```python
from build123d import *

# Parameters (mm, degrees)
F0_W     = 31.8
F0_H     = 15.8
F0_W_2   = 29.4
F0_H_2   = 13.4
F0_R     = 3.25
F0_R_2   = 2.4
F1_DEPTH = 9.6
F2_DEPTH = 7.9
F3_R     = 2.4
F4_DEPTH = 1.7
F5_W     = 0.6
F5_H     = 0.3
F5_W_2   = 0.3
F5_H_2   = 0.6
F6_DEPTH = 7.9


# Not quite as in the source:
# - a feature names something its author has since deleted; it is built from what else it names


with BuildPart() as f1:
    # F0 (on Top) → F1 (new body)
    with BuildSketch(Plane.XY):
        Rectangle(F0_W, F0_H)
        Rectangle(F0_W_2, F0_H_2, mode=Mode.SUBTRACT)
        Rectangle(F0_W_2, F0_H_2)
        with Locations((-8, 0)):
            Circle(F0_R, mode=Mode.SUBTRACT)
        Circle(F0_R, mode=Mode.SUBTRACT)
        with Locations((8, 0)):
            Circle(F0_R, mode=Mode.SUBTRACT)
        with Locations((-8, 0)):
            Circle(F0_R)
        with Locations((-8, 0)):
            Circle(F0_R_2, mode=Mode.SUBTRACT)
        Circle(F0_R)
        Circle(F0_R_2, mode=Mode.SUBTRACT)
        with Locations((8, 0)):
            Circle(F0_R)
        with Locations((8, 0)):
            Circle(F0_R_2, mode=Mode.SUBTRACT)
        with Locations((-8, 0)):
            Circle(F0_R_2)
        Circle(F0_R_2)
        with Locations((8, 0)):
            Circle(F0_R_2)
    extrude(amount=F1_DEPTH)

    # F0 (on Top) → F2 (cut)
    with BuildSketch(Plane.XY):
        Rectangle(F0_W_2, F0_H_2)
        with Locations((-8, 0)):
            Circle(F0_R, mode=Mode.SUBTRACT)
        Circle(F0_R, mode=Mode.SUBTRACT)
        with Locations((8, 0)):
            Circle(F0_R, mode=Mode.SUBTRACT)
        with Locations((-8, 0)):
            Circle(F0_R_2)
        with Locations((8, 0)):
            Circle(F0_R_2)
        Circle(F0_R_2)
    extrude(amount=F2_DEPTH, mode=Mode.SUBTRACT)

    # F3 (on face) → F4 (join)
    with BuildSketch(Plane.XY.offset(9.6)):
        with Locations((-12, 4)):
            Circle(F3_R)
        with Locations((-12, -4)):
            Circle(F3_R)
        with Locations((-4, 4)):
            Circle(F3_R)
        with Locations((-4, -4)):
            Circle(F3_R)
        with Locations((4, 4)):
            Circle(F3_R)
        with Locations((4, -4)):
            Circle(F3_R)
        with Locations((12, 4)):
            Circle(F3_R)
        with Locations((12, -4)):
            Circle(F3_R)
    extrude(amount=F4_DEPTH)

    # F5 (on Top) → F6 (join, through all)
    with BuildSketch(Plane.XY):
        with Locations((-12, -6.55)):
            Rectangle(F5_W, F5_H)
        with Locations((-4, -6.55)):
            Rectangle(F5_W, F5_H)
        with Locations((-14.55, -4)):
            Rectangle(F5_W_2, F5_H_2)
        with Locations((4, -6.55)):
            Rectangle(F5_W, F5_H)
        with Locations((12, -6.55)):
            Rectangle(F5_W, F5_H)
        with Locations((14.55, -4)):
            Rectangle(F5_W_2, F5_H_2)
        with Locations((-4, 6.55)):
            Rectangle(F5_W, F5_H)
        with Locations((14.55, 4)):
            Rectangle(F5_W_2, F5_H_2)
        with Locations((12, 6.55)):
            Rectangle(F5_W, F5_H)
        with Locations((-12, 6.55)):
            Rectangle(F5_W, F5_H)
        with Locations((-14.55, 4)):
            Rectangle(F5_W_2, F5_H_2)
        with Locations((4, 6.55)):
            Rectangle(F5_W, F5_H)
    extrude(amount=F6_DEPTH)


solid = f1.part
```
Geometry check sheet. Reference: the model listing, model coordinates, mm. A direction names the side the tool comes from. Round coordinates to 2 decimals unless told otherwise and drop trailing zeros. Order: outer loops, then holes, each group sorted by start corner. A loop starts at its lowest first (then second) coordinate and runs counter-clockwise, first axis right, second up. Notation, with made-up numbers: M -8.5,70 L 34.5,70 A29 ccw 34.5,106 Z; hole C 13,45.5 d2. An arc over 180 degrees is marked long. Answer as CSV lines item,"result".
1) Tool access check on faces 1 (the face through (-14.398, 4.106, 10.438)), 2 (the face through (0, 7.9, 5)), 3 (the face through (0, 0, 7.9)). Record the directions out of +Z, -Z, +X, -X, +Y, -Y that give a thin tool (end or side, any length) a straight path to the whole face; none if there is none.
Entries:
face 1,"+Z"
face 2,"+Z, -Z, +X, -X, +Y"
face 3,"-Z"
2) Sectioned sample at C-C on z = 1.5. Give the number of separate pieces and of enclosed holes in the cut face, and give its area (3 significant figures).
Entries:
separate pieces,"4"
enclosed holes,"4"
area,"156 mm2"
3) Sectioned sample at D-D on y = -4. Record the cut outline in (x, z).
Entries:
outline,"M -15.9,0 L -14.4,0 L -14.4,7.9 L 14.4,7.9 L 14.4,0 L 15.9,0 L 15.9,9.6 L 14.4,9.6 L 14.4,11.3 L 9.6,11.3 L 9.6,9.6 L 6.4,9.6 L 6.4,11.3 L 1.6,11.3 L 1.6,9.6 L -1.6,9.6 L -1.6,11.3 L -6.4,11.3 L -6.4,9.6 L -9.6,9.6 L -9.6,11.3 L -14.4,11.3 L -14.4,9.6 L -15.9,9.6 Z"
4) Thickness scan on probe 1 along Y at (x, z) = (-8, 3.5); probe 2 along Y at (x, z) = (11.5, 5); probe 3 along X at (y, z) = (-4.5, 7). Record the ranges inside material, lowest first. Write a range as [from, to].
Entries:
probe 1,"[-7.9, -6.7], [-3.25, -2.4], [2.4, 3.25], [6.7, 7.9]"
probe 2,"[-7.9, -6.7], [6.7, 7.9]"
probe 3,"[-15.9, -14.7], [14.7, 15.9]"
5) Gauge pin test, flat end, axial feed: pin 1 Ø1.4 at (x, y) = (8.5, -0.5) entering from -Z. Record the tip position at first contact, or that the pin passes through.
Entries:
pin 1,"z = 7.9"
6) Mould release check, pull along X, two halves, no side actions. Record for faces 4 (the face through (-12, 4, 11.3)), 5 (the face through (-2.579, -1.978, 3.895)): +X half, -X half, draft (parallel to the pull), parting line (faces both ways), or undercut.
Entries:
face 4,"draft"
face 5,"undercut"
7) Sectioned sample at A-A on z = 10.25. Record the cut outline in (x, y), and give its area (3 significant figures).
Entries:
outline,"C -12,-4 d4.8; C -12,4 d4.8; C -4,-4 d4.8; C -4,4 d4.8; C 4,-4 d4.8; C 4,4 d4.8; C 12,-4 d4.8; C 12,4 d4.8"
area,"145 mm2"
8) Sectioned sample at B-B on x = 4. Record the cut outline in (y, z), and give its area (3 significant figures).
Entries:
outline,"M -7.9,0 L -6.4,0 L -6.4,7.9 L 6.4,7.9 L 6.4,0 L 7.9,0 L 7.9,9.6 L 6.4,9.6 L 6.4,11.3 L 1.6,11.3 L 1.6,9.6 L -1.6,9.6 L -1.6,11.3 L -6.4,11.3 L -6.4,9.6 L -7.9,9.6 Z"
area,"66.9 mm2"
